Autodesk Inventor part; units mm, degrees
ref_plane "YZ Plane" through (0, 0, 0) normal (1, 0, 0) x (0, 1, 0)
ref_plane "XZ Plane" through (0, 0, 0) normal (0, 1, 0) x (-1, 0, 0)
ref_plane "XY Plane" through (0, 0, 0) normal (0, 0, 1) x (1, 0, 0)
sketch "Sketch2" plane through (0, 0, 0) normal (0, 0, 1) x (1, 0, 0)
  line L0 (20.59, 130) -> (59.7544, 117.2747)
  line L1 (59.7544, 117.2747) -> (93.0697, 93.0697)
  line L2 (93.0697, 93.0697) -> (117.2747, 59.7544)
  line L3 (117.2747, 59.7544) -> (130, 20.59)
  line L4 (130, 20.59) -> (130, -20.59)
  line L5 (130, -20.59) -> (117.2747, -59.7544)
  line L6 (117.2747, -59.7544) -> (93.0697, -93.0697)
  line L7 (93.0697, -93.0697) -> (59.7544, -117.2747)
  line L8 (59.7544, -117.2747) -> (20.59, -130)
  line L9 (20.59, -130) -> (-20.59, -130)
  line L10 (-20.59, -130) -> (-59.7544, -117.2747)
  line L11 (-59.7544, -117.2747) -> (-93.0697, -93.0697)
  line L12 (-93.0697, -93.0697) -> (-117.2747, -59.7544)
  line L13 (-117.2747, -59.7544) -> (-130, -20.59)
  line L14 (-130, -20.59) -> (-130, 20.59)
  line L15 (-130, 20.59) -> (-117.2747, 59.7544)
  line L16 (-117.2747, 59.7544) -> (-93.0697, 93.0697)
  line L17 (-93.0697, 93.0697) -> (-59.7544, 117.2747)
  line L18 (-59.7544, 117.2747) -> (-20.59, 130)
  line L19 (-20.59, 130) -> (20.59, 130)
  circle A0 centre (0, 0) radius 8
  point P0 (0, 130)
  dimension "d0" = 260
  dimension "d3" = 16
extrude "Extrusion1" add sketch "Sketch2" along normal blind 50
sketch "Sketch3" plane through (0, 0, 50) normal (0, 0, 1) x (1, 0, 0)
  circle A0 centre (0, 0) radius 8
  line L0 (14.4338, 25) -> (28.8675, 0)
  line L1 (28.8675, 0) -> (14.4338, -25)
  line L2 (14.4338, -25) -> (-14.4338, -25)
  line L3 (-14.4338, -25) -> (-28.8675, 0)
  line L4 (-28.8675, 0) -> (-14.4338, 25)
  line L5 (-14.4338, 25) -> (14.4338, 25)
  point P0 (0, 25)
  dimension "d4" = 50
extrude "Extrusion2" cut sketch "Sketch3" against normal blind 16
properties part number "PropellerHub"
Design review of the part built by this model. Coordinates are the model's own, in mm. A direction names the side the tool comes from. Coordinates: 2 decimals unless noted, no trailing zeros. Order: outer loops, then holes, each group sorted by start corner. A loop starts at its lowest first (then second) coordinate and runs counter-clockwise, first axis right, second up.
Item 1: Take a section at D-D, the plane x = -89. Write out the cut boundary in (y, z).
Item 2: The part is to be moulded in two halves that separate along Y. For faces 3 (the flat face through (40.446, -123.548, 24.65)), 4 (the flat face through (6, 6, 34)), 5 (the flat face through (-21.75, 12.33, 42.11)), 6 (the flat face through (-123.726, 39.898, 24.65)), say which applies: pulls with the +Y half, pulls with the -Y half, needs draft (parallel to the pull), parting line crosses it, or undercut.
Item 3: Take a section at C-C, the plane y = 103.5. Write out the cut boundary in (x, z).
Item 4: For line 1 (Y direction, x = 0, z = 17); line 2 (Z direction, x = 9.5, y = 17); line 3 (Y direction, x = -25.5, z = 47), list the stretches that pass through material, from the lowest coordinate up.
Item 5: Take a section at B-B, the plane z = 37.5. Write out the cut boundary in (x, y), then the cut area to 3 significant figures.
Item 6: For pin 1 Ø2 at (y, z) = (-54, 16) entering from +X; pin 2 Ø5 at (y, z) = (-77, 5.5) entering from +X; pin 3 Ø12 at (y, z) = (-94, 30) entering from -X; pin 4 Ø14.5 at (x, y) = (0, 0) entering from -Z, all flat-tipped, find the tip position at first contact; note any pin that passes through.
Item 7: For faces 1 (the flat face through (21.75, -12.33, 42.11)), 2 (the flat face through (-123.548, -40.446, 24.65)), list the 3-axis set-ups (+Z, -Z, +X, -X, +Y, -Y) from which the entire face can be reached by the end or side of a thin tool; tool diameter is ignored.
Item 8: Take a section at A-A, the plane x = 0. Write out the cut boundary in (y, z), then the cut area to 3 significant figures.
The answers:
1. outline: (-96.03, 0) - (96.03, 0) - (96.03, 50) - (-96.03, 50) - close
2. face 3: pulls with the -Y half
2. face 4: undercut
2. face 5: undercut
2. face 6: pulls with the +Y half
3. outline: (-78.71, 0) - (78.71, 0) - (78.71, 50) - (-78.71, 50) - close
4. line 1: y = -130 to -8, 8 to 130
4. line 2: z = 0 to 34
4. line 3: y = -128.4 to -5.83, 5.83 to 128.4
5. outline: (-130, -20.59) - (-117.27, -59.75) - (-93.07, -93.07) - (-59.75, -117.27) - (-20.59, -130) - (20.59, -130) - (59.75, -117.27) - (93.07, -93.07) - (117.27, -59.75) - (130, -20.59) - (130, 20.59) - (117.27, 59.75) - (93.07, 93.07) - (59.75, 117.27) - (20.59, 130) - (-20.59, 130) - (-59.75, 117.27) - (-93.07, 93.07) - (-117.27, 59.75) - (-130, 20.59) - close; hole (-28.87, 0) - (-14.43, -25) - (14.43, -25) - (28.87, 0) - (14.43, 25) - (-14.43, 25) - close
5. area: 51,400 mm2
6. pin 1: stops at x = 119.47
6. pin 2: stops at x = 106.56
6. pin 3: stops at x = -96.75
6. pin 4: passes through
7. face 1: +Z
7. face 2: +Z, -Z, -X, -Y
8. outline: (-130, 0) - (-8, 0) - (-8, 34) - (-25, 34) - (-25, 50) - (-130, 50) - close; (8, 0) - (130, 0) - (130, 50) - (25, 50) - (25, 34) - (8, 34) - close
8. area: 11,700 mm2
